Verification items for the finished model (mm, model axes). A direction names the side the tool comes from. Give positions to 0.01 mm unless a question says otherwise; leave off trailing zeros. Order: outer loops, then holes, each group sorted by start corner. A loop starts at its lowest first (then second) coordinate and runs counter-clockwise, first axis right, second up.
from build123d import *

# Parameters (mm, degrees)
SKELTON_BASE_DEPTH = 2
SKETCH3_R          = 2.05
SKETCH3_R_2        = 0.75
SUPPORT_LEG_DEPTH  = 20
SKETCH5_R          = 3.5
SKETCH5_R_2        = 1.25
SKETCH5_R_3        = 1.247534176
SUPPORT_HEAD_DEPTH = 1.5


with BuildPart() as part:
    # skelton_drawing → Skelton_base (new body)
    with BuildSketch(Plane(origin=(0, 0, 0), x_dir=(1, 0, 0), z_dir=(0, 1, 0))):
        with BuildLine():
            Line((15.163755459, 7.25), (15.163755459, -7.25))
            ThreePointArc((15.163755459, -7.25), (15.090532154, -7.426776695), (14.913755459, -7.5))
            Line((14.913755459, -7.5), (10.663755459, -7.5))
            Line((10.663755459, -7.5), (10.663755459, -13.511910465))
            ThreePointArc((10.663755459, -13.511910465), (10.163755459, -17.55), (9.663755459, -13.511910465))
            Line((9.663755459, -13.511910465), (9.663755459, -7.5))
            Line((9.663755459, -7.5), (5.413755459, -7.5))
            ThreePointArc((5.413755459, -7.5), (5.236978763, -7.426776695), (5.163755459, -7.25))
            Line((5.163755459, -7.25), (5.163755459, -0.5))
            Line((5.163755459, -0.5), (3.075114856, -0.5))
            ThreePointArc((3.075114856, -0.5), (2.898338161, -0.573223305), (2.825114856, -0.75))
            Line((2.825114856, -0.75), (2.825114856, -14.75))
            ThreePointArc((2.825114856, -14.75), (2.605444942, -15.280330086), (2.075114856, -15.5))
            Line((2.075114856, -15.5), (-0.424885144, -15.5))
            ThreePointArc((-0.424885144, -15.5), (-0.95521523, -15.280330086), (-1.174885144, -14.75))
            Line((-1.174885144, -14.75), (-1.174885144, 14.5))
            Line((-1.174885144, 14.5), (-3.174885144, 14.5))
            Line((-3.174885144, 14.5), (-3.174885144, -14.75))
            ThreePointArc((-3.174885144, -14.75), (-3.394555058, -15.280330086), (-3.924885144, -15.5))
            Line((-3.924885144, -15.5), (-6.424885144, -15.5))
            ThreePointArc((-6.424885144, -15.5), (-6.95521523, -15.280330086), (-7.174885144, -14.75))
            Line((-7.174885144, -14.75), (-7.174885144, 14.5))
            Line((-7.174885144, 14.5), (-9.174885144, 14.5))
            Line((-9.174885144, 14.5), (-9.174885144, -14.75))
            ThreePointArc((-9.174885144, -14.75), (-9.394555058, -15.280330086), (-9.924885144, -15.5))
            Line((-9.924885144, -15.5), (-12.424885144, -15.5))
            ThreePointArc((-12.424885144, -15.5), (-12.95521523, -15.280330086), (-13.174885144, -14.75))
            Line((-13.174885144, -14.75), (-13.174885144, -0.5))
            Line((-13.174885144, -0.5), (-19.274885144, -0.5))
            Line((-19.274885144, -0.5), (-21.674885144, -2.5))
            Line((-21.674885144, -2.5), (-26.674885144, -2.5))
            Line((-26.674885144, -2.5), (-29.074885144, -0.5))
            Line((-29.074885144, -0.5), (-33.68175141, -0.5))
            ThreePointArc((-33.68175141, -0.5), (-33.777422268, -0.519030117), (-33.858528105, -0.573223305))
            Line((-33.858528105, -0.573223305), (-37.712081496, -4.426776695))
            ThreePointArc((-37.712081496, -4.426776695), (-37.793187333, -4.480969883), (-37.888858191, -4.5))
            Line((-37.888858191, -4.5), (-45.742411582, -4.5))
            ThreePointArc((-45.742411582, -4.5), (-45.919188277, -4.573223305), (-45.992411582, -4.75))
            Line((-45.992411582, -4.75), (-45.992411582, -7.440983006))
            ThreePointArc((-45.992411582, -7.440983006), (-46.492411582, -8.75), (-46.992411582, -7.440983006))
            Line((-46.992411582, -7.440983006), (-46.992411582, -4.5))
            Line((-46.992411582, -4.5), (-49.992411582, -4.5))
            Line((-49.992411582, -4.5), (-49.992411582, -7.440983006))
            ThreePointArc((-49.992411582, -7.440983006), (-50.492411582, -8.75), (-50.992411582, -7.440983006))
            Line((-50.992411582, -7.440983006), (-50.992411582, -4.25))
            ThreePointArc((-50.992411582, -4.25), (-50.772741668, -3.719669914), (-50.242411582, -3.5))
            Line((-50.242411582, -3.5), (-38.303071753, -3.5))
            ThreePointArc((-38.303071753, -3.5), (-38.207400895, -3.480969883), (-38.126295058, -3.426776695))
            Line((-38.126295058, -3.426776695), (-34.876295058, -0.176776695))
            ThreePointArc((-34.876295058, -0.176776695), (-34.803071753, 0), (-34.876295058, 0.176776695))
            Line((-34.876295058, 0.176776695), (-38.126295058, 3.426776695))
            ThreePointArc((-38.126295058, 3.426776695), (-38.207400895, 3.480969883), (-38.303071753, 3.5))
            Line((-38.303071753, 3.5), (-46.242411582, 3.5))
            Line((-46.242411582, 3.5), (-50.242411582, 3.5))
            ThreePointArc((-50.242411582, 3.5), (-50.772741668, 3.719669914), (-50.992411582, 4.25))
            Line((-50.992411582, 4.25), (-50.992411582, 7.440983006))
            ThreePointArc((-50.992411582, 7.440983006), (-50.492411582, 8.75), (-49.992411582, 7.440983006))
            Line((-49.992411582, 7.440983006), (-49.992411582, 4.5))
            Line((-49.992411582, 4.5), (-46.992411582, 4.5))
            Line((-46.992411582, 4.5), (-46.992411582, 7.440983006))
            ThreePointArc((-46.992411582, 7.440983006), (-46.492411582, 8.75), (-45.992411582, 7.440983006))
            Line((-45.992411582, 7.440983006), (-45.992411582, 4.75))
            ThreePointArc((-45.992411582, 4.75), (-45.919188277, 4.573223305), (-45.742411582, 4.5))
            Line((-45.742411582, 4.5), (-37.888858191, 4.5))
            ThreePointArc((-37.888858191, 4.5), (-37.793187333, 4.480969883), (-37.712081496, 4.426776695))
            Line((-37.712081496, 4.426776695), (-33.858528105, 0.573223305))
            ThreePointArc((-33.858528105, 0.573223305), (-33.777422268, 0.519030117), (-33.68175141, 0.5))
            Line((-33.68175141, 0.5), (-29.074885144, 0.5))
            Line((-29.074885144, 0.5), (-26.674885144, 2.5))
            Line((-26.674885144, 2.5), (-21.674885144, 2.5))
            Line((-21.674885144, 2.5), (-19.274885144, 0.5))
            Line((-19.274885144, 0.5), (-12.924885144, 0.5))
            ThreePointArc((-12.924885144, 0.5), (-12.394555058, 0.280330086), (-12.174885144, -0.25))
            Line((-12.174885144, -0.25), (-12.174885144, -14.5))
            Line((-12.174885144, -14.5), (-10.174885144, -14.5))
            Line((-10.174885144, -14.5), (-10.174885144, 14.75))
            ThreePointArc((-10.174885144, 14.75), (-9.95521523, 15.280330086), (-9.424885144, 15.5))
            Line((-9.424885144, 15.5), (-6.924885144, 15.5))
            ThreePointArc((-6.924885144, 15.5), (-6.394555058, 15.280330086), (-6.174885144, 14.75))
            Line((-6.174885144, 14.75), (-6.174885144, -14.5))
            Line((-6.174885144, -14.5), (-4.174885144, -14.5))
            Line((-4.174885144, -14.5), (-4.174885144, 14.75))
            ThreePointArc((-4.174885144, 14.75), (-3.95521523, 15.280330086), (-3.424885144, 15.5))
            Line((-3.424885144, 15.5), (-0.924885144, 15.5))
            ThreePointArc((-0.924885144, 15.5), (-0.394555058, 15.280330086), (-0.174885144, 14.75))
            Line((-0.174885144, 14.75), (-0.174885144, -14.5))
            Line((-0.174885144, -14.5), (1.825114856, -14.5))
            Line((1.825114856, -14.5), (1.825114856, 0.25))
            ThreePointArc((1.825114856, 0.25), (1.898338161, 0.426776695), (2.075114856, 0.5))
            Line((2.075114856, 0.5), (5.163755459, 0.5))
            Line((5.163755459, 0.5), (5.163755459, 7.25))
            ThreePointArc((5.163755459, 7.25), (5.236978763, 7.426776695), (5.413755459, 7.5))
            Line((5.413755459, 7.5), (9.663755459, 7.5))
            Line((9.663755459, 7.5), (9.663755459, 13.511910465))
            ThreePointArc((9.663755459, 13.511910465), (10.163755459, 17.55), (10.663755459, 13.511910465))
            Line((10.663755459, 13.511910465), (10.663755459, 7.5))
            Line((10.663755459, 7.5), (14.913755459, 7.5))
            ThreePointArc((14.913755459, 7.5), (15.090532154, 7.426776695), (15.163755459, 7.25))
        make_face()
    extrude(amount=SKELTON_BASE_DEPTH)

    # Sketch3 → Support_leg (add)
    with BuildSketch(Plane(origin=(0, 2, 0), x_dir=(1, 0, 0), z_dir=(0, 1, 0))):
        with Locations(Location((10.163755459, 15.5, 0), (0, 0, 255.883019429))):
            Circle(SKETCH3_R)
        with Locations(Location((10.163755459, -15.5, 0), (0, 0, 75.883019429))):
            Circle(SKETCH3_R)
        with Locations(Location((-46.492411582, 8, 0), (0, 0, 228.189685104))):
            Circle(SKETCH3_R_2)
        with Locations(Location((-50.492411582, 8, 0), (0, 0, 311.810314896))):
            Circle(SKETCH3_R_2)
        with Locations(Location((-46.492411582, -8, 0), (0, 0, 48.189685104))):
            Circle(SKETCH3_R_2)
        with Locations(Location((-50.492411582, -8, 0), (0, 0, 48.189685104))):
            Circle(SKETCH3_R_2)
    extrude(amount=SUPPORT_LEG_DEPTH)

    # Sketch5 → Support_head (add)
    with BuildSketch(Plane(origin=(0, 22, 0), x_dir=(1, 0, 0), z_dir=(0, 1, 0))):
        with Locations(Location((10.163755459, -15.5, 0), (0, 0, 270))):
            Circle(SKETCH5_R)
        with Locations(Location((10.163755459, 15.5, 0), (0, 0, 270))):
            Circle(SKETCH5_R)
        with Locations(Location((-46.492411582, 8, 0), (0, 0, 270))):
            Circle(SKETCH5_R_2)
        with Locations(Location((-50.492411582, 8, 0), (0, 0, 270))):
            Circle(SKETCH5_R_2)
        with Locations(Location((-46.492411582, -8, 0), (0, 0, 270))):
            Circle(SKETCH5_R_2)
        with Locations(Location((-50.492411582, -8, 0), (0, 0, 270))):
            Circle(SKETCH5_R_3)
    extrude(amount=SUPPORT_HEAD_DEPTH)


solid = part.part
(1) Scan lines: line 1 (X direction, y = 18.5, z = 8); line 2 (Y direction, x = 8.5, z = 14); line 3 (Y direction, x = 7.5, z = 1.5). Record each from-to range of solid material in increasing order.
Solved:
line 1: x = -51.24 to -49.74, -47.24 to -45.74
line 2: y = 22 to 23.5
line 3: y = 0 to 2
(2) Section check C-C, the plane x = 9. Enter the section's corners in (y, z).
Solved:
outline: (0, -17.19) - (22, -17.19) - (22, -18.8) - (23.5, -18.8) - (23.5, -12.2) - (22, -12.2) - (22, -13.81) - (0, -13.81) - close; (0, -7.5) - (2, -7.5) - (2, 7.5) - (0, 7.5) - close; (0, 13.81) - (22, 13.81) - (22, 12.2) - (23.5, 12.2) - (23.5, 18.8) - (22, 18.8) - (22, 17.19) - (0, 17.19) - close
(3) Go/stop test with flat-tipped pins: pin 1 (1 mm diameter, centred on x = -48.5, y = 1, fed in from +Z); pin 2 (0.6 mm diameter, centred on y = 1.5, z = -6.5, fed in from -X); pin 3 (1 mm diameter, centred on x = -15, y = 1, fed in from +Z). Record where each tip stops, or that it passes through.
Solved:
pin 1: stops at z = 4.5
pin 2: stops at x = -50.99
pin 3: stops at z = 0.5
(4) Section check A-A, the plane z = 10. Enter the section's corners in (x, y), then the cut area to 3 significant figures.
Solved:
outline: (-13.17, 0) - (-12.17, 0) - (-12.17, 2) - (-13.17, 2) - close; (-10.17, 0) - (-9.17, 0) - (-9.17, 2) - (-10.17, 2) - close; (-7.17, 0) - (-6.17, 0) - (-6.17, 2) - (-7.17, 2) - close; (-4.17, 0) - (-3.17, 0) - (-3.17, 2) - (-4.17, 2) - close; (-1.17, 0) - (-0.17, 0) - (-0.17, 2) - (-1.17, 2) - close; (1.83, 0) - (2.83, 0) - (2.83, 2) - (1.83, 2) - close; (9.66, 0) - (10.66, 0) - (10.66, 2) - (9.66, 2) - close
area: 14.0 mm2
(5) Release check for a two-part mould opening along Z. For faces 1 (the flat face through (-50.992, 1, 6)), 2 (the flat face through (-7.175, 1, 0)), 3 (the flat face through (-35.812, 0.986, -2.527)) record: pulls with the +Z half, pulls with the -Z half, needs draft (parallel to the pull), parting line crosses it, or undercut.
Solved:
face 1: undercut
face 2: needs draft
face 3: pulls with the -Z half
(6) Section check B-B, the plane y = 17. Enter the section's corners in (x, z).
Solved:
outline: circle Ø1.5 at (-50.49, -8); circle Ø1.5 at (-50.49, 8); circle Ø1.5 at (-46.49, -8); circle Ø1.5 at (-46.49, 8); circle Ø4.1 at (10.16, -15.5); circle Ø4.1 at (10.16, 15.5)
(7) Section check D-D, the plane z = -1.5. Enter the section's corners in (x, y), then the cut area to 3 significant figures.
Solved:
outline: (-36.2, 0) - (-34.79, 0) - (-34.79, 2) - (-36.2, 2) - close; (-27.87, 0) - (-20.47, 0) - (-20.47, 2) - (-27.87, 2) - close; (-10.17, 0) - (-9.17, 0) - (-9.17, 2) - (-10.17, 2) - close; (-7.17, 0) - (-6.17, 0) - (-6.17, 2) - (-7.17, 2) - close; (-4.17, 0) - (-3.17, 0) - (-3.17, 2) - (-4.17, 2) - close; (-1.17, 0) - (-0.17, 0) - (-0.17, 2) - (-1.17, 2) - close; (5.16, 0) - (15.16, 0) - (15.16, 2) - (5.16, 2) - close
area: 45.6 mm2
(8) Set-up check for faces 4 (the flat face through (-8, 1, -14.5)), 5 (the flat face through (-12.175, 1, 7)), 6 (the flat face through (13, 1, -7.5)): record each of +Z, -Z, +X, -X, +Y, -Y from which the full face is reachable in a straight line by a thin tool's end or side.
Solved:
face 4: +Z, +Y, -Y
face 5: -Z, +Y, -Y
face 6: +X, +Y, -Y
